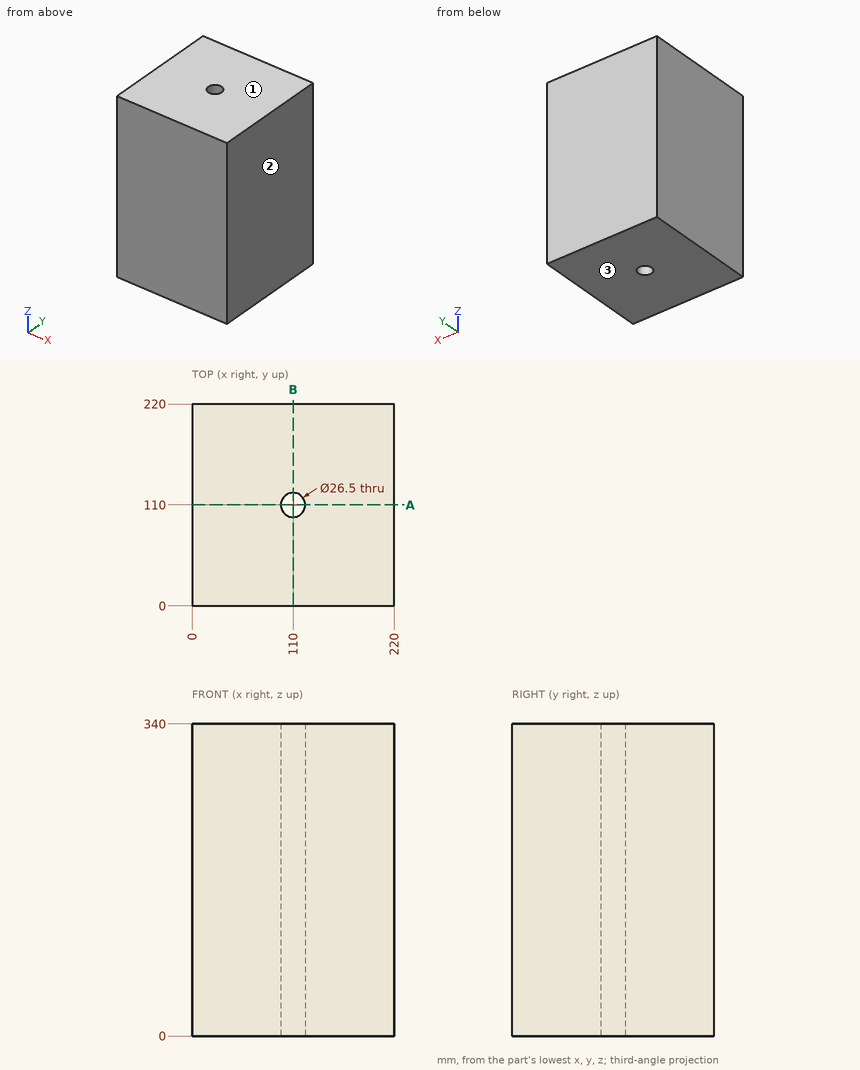
Here's the drawing with two shaded views (mm, measured from the low corner). I have some questions. Give positions to 0.01 mm unless a question says otherwise; leave off trailing zeros. Order: outer loops, then holes, each group sorted by start corner. A loop starts at its lowest first (then second) coordinate and runs counter-clockwise, first axis right, second up. Notation, with made-up numbers: (-31, 19) -> (-24, 19) arc R22 ccw to (-24, 58) -> close; hole circle Ø10 at (68, -7). An arc over 180 degrees is marked (long way). One line per item, written item: value. Start each with the question number.
1. I need wall thicknesses on probe 1 along Y at (x, z) = (110, 182). Which ranges of the line are inside material? Lowest first, please. Write a range as from..to.
2. We'd pull the mould along Z, two halves only. Please class the marked faces 1, 2 and 3: released by +Z, released by -Z, zero draft, split by the parting line, or undercut.
3. Imagine slicing it at A-A, the plane y = 110. List the corners of the cut face in (x, z) for me, plus the area to 3 significant figures.
4. Will this pin go through, and if not, where does the flat tip stop? pin 1 Ø16 at (x, y) = (110, 110) entering from +Z.
Values follow:
1. probe 1: y = 0..96.75, 123.25..220
2. face 1: released by +Z
2. face 2: zero draft
2. face 3: released by -Z
3. outline: (0, 0) -> (96.75, 0) -> (96.75, 340) -> (0, 340) -> close; (123.25, 0) -> (220, 0) -> (220, 340) -> (123.25, 340) -> close
3. area: 65,800 mm2
4. pin 1: passes through
